from build123d import *

# Parameters (mm, degrees)
F0_W     = 10
F0_H     = 10
F0_W_2   = 30
F1_DEPTH = 70
F2_W     = 10
F2_H     = 10
F2_W_2   = 30
F2_H_2   = 30
F3_DEPTH = 100


with BuildPart() as f1:
    # F0 (on Front) → F1 (new body)
    with BuildSketch(Plane.XZ):
        Polygon((-15, 70), (-25, 70), (-25, 60), (-35, 60), (-35, 50), (-25, 50), (-25, 40), (-35, 40), (-35, 30), (-25, 30), (-25, 20), (-35, 20), (-35, -10), (-25, -10), (-25, -20), (-35, -20), (-35, -30), (-25, -30), (-25, -40), (-35, -40), (-35, -70), (-5, -70), (-5, -40), (-15, -40), (-15, -30), (15, -30), (15, -40), (5, -40), (5, -70), (35, -70), (35, -40), (25, -40), (25, -30), (35, -30), (35, -20), (25, -20), (25, -10), (35, -10), (35, 20), (25, 20), (25, 30), (35, 30), (35, 40), (25, 40), (25, 50), (35, 50), (35, 60), (25, 60), (25, 70), (15, 70), (15, 60), (-15, 60), align=None)
        with Locations((-20, -55)):
            Rectangle(F0_W, F0_H, mode=Mode.SUBTRACT)
        with Locations((20, -55)):
            Rectangle(F0_W, F0_H, mode=Mode.SUBTRACT)
        with Locations((-20, 5)):
            Rectangle(F0_W, F0_H, mode=Mode.SUBTRACT)
        Polygon((-5, -10), (-5, 20), (-15, 20), (-15, 30), (15, 30), (15, 20), (5, 20), (5, -10), (15, -10), (15, -20), (-15, -20), (-15, -10), align=None, mode=Mode.SUBTRACT)
        with Locations((20, 5)):
            Rectangle(F0_W, F0_H, mode=Mode.SUBTRACT)
        with Locations((0, 45)):
            Rectangle(F0_W_2, F0_H, mode=Mode.SUBTRACT)
    extrude(amount=F1_DEPTH)

    # F2 (on face) → F3 (cut)
    with BuildSketch(Plane.YZ.offset(35)):
        Polygon((-20, 30), (-50, 30), (-50, 20), (-40, 20), (-40, -10), (-50, -10), (-50, -20), (-20, -20), (-20, -10), (-30, -10), (-30, 20), (-20, 20), align=None)
        with Locations((-5, -15)):
            Rectangle(F2_W, F2_H)
        with Locations((-15, 5)):
            Rectangle(F2_W, F2_H)
        with Locations((-55, 5)):
            Rectangle(F2_W, F2_H)
        with Locations((-65, 25)):
            Rectangle(F2_W, F2_H)
        with Locations((-5, 25)):
            Rectangle(F2_W, F2_H)
        with Locations((-5, 45)):
            Rectangle(F2_W, F2_H)
        with Locations((-35, 45)):
            Rectangle(F2_W_2, F2_H)
        with Locations((-65, 45)):
            Rectangle(F2_W, F2_H)
        with Locations((-65, 65)):
            Rectangle(F2_W, F2_H)
        with Locations((-35, 65)):
            Rectangle(F2_W_2, F2_H)
        with Locations((-5, 65)):
            Rectangle(F2_W, F2_H)
        with Locations((-65, -15)):
            Rectangle(F2_W, F2_H)
        with Locations((-65, -35)):
            Rectangle(F2_W, F2_H)
        Polygon((-40, -40), (-30, -40), (-20, -40), (-20, -30), (-50, -30), (-50, -40), align=None)
        with Locations((-5, -35)):
            Rectangle(F2_W, F2_H)
        with Locations((-15, -55)):
            Rectangle(F2_W, F2_H)
        with Locations((-55, -55)):
            Rectangle(F2_W, F2_H)
        with Locations((-35, -55)):
            Rectangle(F2_W, F2_H_2)
    extrude(amount=-F3_DEPTH, mode=Mode.SUBTRACT)


solid = f1.part
Here's how the part is built. I have some questions about the finished solid (model axes, mm). A direction names the side the tool comes from. Round coordinates to 2 decimals unless told otherwise and drop trailing zeros. Write each loop counter-clockwise with the first axis right and the second up, starting at its lowest first coordinate (ties: lowest second). Pieces come first, ordered by that corner, then holes. Notation, with made-up numbers: (62, -3.5) -> (109, -3.5) arc R11 cw to (109, 17.5) -> close; hole circle Ø7 at (29, -21.75). An arc over 180 degrees is marked (long way). One line per item, written item: value.
1) Suppose I cut it at A-A on y = -34.5. List the corners of the cut face in (x, z) for me, plus the area to 3 significant figures.
Filled sheet:
outline: (-35, -30) -> (35, -30) -> (35, -20) -> (-35, -20) -> close; (-35, 30) -> (35, 30) -> (35, 40) -> (-35, 40) -> close; (-35, 50) -> (35, 50) -> (35, 60) -> (-35, 60) -> close
area: 2,100 mm2
2) We'd pull the mould along X, two halves only. Please class faces 1 (the face through (-20, -50, 25)), 2 (the face through (-25, -55, -15)), 3 (the face through (0, -35, 30)): released by +X, released by -X, zero draft, split by the parting line, or undercut.
Filled sheet:
face 1: zero draft
face 2: released by -X
face 3: undercut
3) For faces 4 (the face through (-20, -55, 10)), 5 (the face through (10, -50, -55)), 6 (the face through (25, -5, -55)), which set-ups out of +Z, -Z, +X, -X, +Y, -Y let a thin tool reach every point of the face, with its end or its side?
Filled sheet:
face 4: none
face 5: +X, -X
face 6: +Y, -Y
4) Suppose I cut it at B-B on x = -19. Give the number of separate pieces and of enclosed holes in the cut face, plus the area to 3 significant figures.
Filled sheet:
separate pieces: 4
enclosed holes: 1
area: 5,500 mm2
5) I'm going to push flat-ended pins straight in: pin 1 Ø10 at (x, y) = (14.5, -36) entering from +Z; pin 2 Ø8 at (y, z) = (-13.5, -14.5) entering from +X; pin 3 Ø5 at (y, z) = (-12.5, 66.5) entering from -X. Where does each tip first touch, or does it pass through?
Filled sheet:
pin 1: stops at z = 60
pin 2: stops at x = 25
pin 3: stops at x = -25
6) If I drill on line 1 (Z direction, x = -27, y = -24); line 2 (Z direction, x = 1.5, y = -55.5); line 3 (Y direction, x = 19.5, z = 21), over which ranges is the centre line in solid material (lowest first)? Write a range as [from, to].
Filled sheet:
line 1: z = [-70, -40], [-30, -20], [-10, 20], [30, 40], [50, 60]
line 2: z = [-30, -20], [30, 40], [50, 60]
line 3: y = [-60, -50], [-20, -10]
7) Suppose I cut it at C-C on z = -43. List the corners of the cut face in (x, y) for me.
Filled sheet:
outline: (-35, -70) -> (-5, -70) -> (-5, -40) -> (-35, -40) -> close; (-35, -30) -> (-5, -30) -> (-5, 0) -> (-35, 0) -> close; (5, -70) -> (35, -70) -> (35, -40) -> (5, -40) -> close; (5, -30) -> (35, -30) -> (35, 0) -> (5, 0) -> close
